Can you work these out from the model? Positions are in its coordinate system, mm. A direction names the side the tool comes from. Coordinates: 2 decimals unless noted, no trailing zeros. Loops run counter-clockwise (first coordinate to the right, second up) from the corner with the lowest first, then second, coordinate; pieces in that order, holes last.
Autodesk Inventor part; units mm, degrees
ref_plane "YZ Plane" through (0, 0, 0) normal (1, 0, 0) x (0, 1, 0)
ref_plane "XZ Plane" through (0, 0, 0) normal (0, 1, 0) x (-1, 0, 0)
ref_plane "XY Plane" through (0, 0, 0) normal (0, 0, 1) x (1, 0, 0)
sketch "Sketch1" plane through (0, 0, 0) normal (0, 0, 1) x (1, 0, 0)
  line L0 (185, -55) -> (-185, -55)
  line L1 (185, 55) -> (-185, 55)
  circle A0 centre (65, -25) radius 5.25
  line L2 (185, 55) -> (185, -55)
  line L3 (-185, 55) -> (-185, -55)
  line L4 (185, 55) -> (-185, -55) construction
  line L5 (185, -55) -> (-185, 55) construction
  line L6 (65, 25) -> (65, -25) construction
  line L7 (152.75, -30.25) -> (157.25, -30.25) construction
  line L8 (152.75, -35.5) -> (157.25, -35.5)
  line L9 (157.25, -25) -> (152.75, -25)
  arc A1 (152.75, -25) -> (152.75, -35.5) centre (152.75, -30.25) ccw
  arc A2 (157.25, -35.5) -> (157.25, -25) centre (157.25, -30.25) ccw
  line L10 (0, 0) -> (155, 0) construction
  line L11 (155, 0) -> (155, -30.25) construction
  dimension "d25" = 50
  dimension "d57" = 2.25
  dimension "d58" = 10.5
  dimension "d59" = 30.25
  dimension "d60" = 155
  dimension "d61" = 110
  dimension "d62" = 370
  dimension "d73" = 65
extrude "Plate1" add sketch "Sketch1" against normal blind 5 contours L0 L3 L1 L2 | A0 | A1 L9 A2 L8
sketch "Sketch4" plane through (185, 50, 0) normal (0, 1, 0) x (-1, 0, 0)
  line L0 (370, 0) -> (0, 0)
  line L1 (0, 0) -> (0, -40)
  line L2 (0, -40) -> (370, -40)
  line L3 (370, -40) -> (370, 0)
edge flange "Flange1" height 40 angle 90 thickness 5 bend radius 5 thickness toward (0, 1, 0) relief tear relief width 5 relief depth 2.5 corner gap 5 corner form 0 edges at (0, 55, -5) (0, -55, -5) wall of the first edge with corners at (-185, 50, 0) (185, 50, 0) (185, 50, -40) (-185, 50, -40)
bend "Bend3"
corner "Corner3"
extrude "Cut1" cut sketch "Sketch1" against normal blind 5 contours A1 L9 A2 L8
extrude "Cut2" cut sketch "Sketch1" against normal blind 5 contours A0
mirror "Mirror1" about plane through (0, 0, 0) normal (0, 1, 0) of "Cut2", "Cut1"
mirror "Mirror2" about plane through (0, 0, 0) normal (1, 0, 0) of "Cut2", "Cut1", "Mirror1"
equation "\"d74\" = Thickness"
equation "\"d76\" = Thickness"
equation "\"d78\" = Thickness"
equation "\"d63\" = BendReliefWidth"
equation "\"d64\" = BendReliefDepth"
equation "\"d65\" = MinimumRemnant"
equation "\"d66\" = BendRadius"
equation "\"d69\" = BendRadius"
equation "\"d70\" = CornerReliefSize"
equation "\"d71\" = GapSize"
equation "\"d72\" = JacobiRadiusSize"
equation "\"BendRadius\" = Thickness"
equation "\"BendReliefWidth\" = Thickness"
equation "\"BendReliefDepth\" = 0.5 * Thickness"
equation "\"TransitionRadius\" = BendRadius"
equation "\"JacobiRadiusSize\" = Thickness"
equation "\"d36\" = BendRadius"
equation "\"GapSize\" = Thickness"
properties part number "ADSK-MH-10032" material "Steel, Mild"
Item 1: I'm going to push flat-ended pins straight in: P1, Ø1.3, axis at x = -155, z = -2.5, coming from the +Y side; P2, Ø5, axis at x = 154.5, z = -3, coming from the +Y side; P3, Ø2, axis at x = -156, z = -2.5, coming from the -Y side. Where does each tip first touch, or does it pass through?
Results are:
P1: stops at y = 52.29
P2: stops at y = 53.93
P3: stops at y = -52.6
Item 2: Suppose I cut it at A-A, the plane z = -23. Please give me the cut outline in (x, y), plus the area to 3 significant figures.
Results are:
outline: (-185, -55) - (185, -55) - (185, -50) - (-185, -50) - close; (-185, 50) - (185, 50) - (185, 55) - (-185, 55) - close
area: 3,700 mm2
Item 3: Suppose I cut it at C-C, the plane x = -116.5. Please give me the cut outline in (y, z).
Results are:
outline: (-55, -40) - (-50, -40) - (-50, -10) arc R5 cw to (-45, -5) - (45, -5) arc R5 cw to (50, -10) - (50, -40) - (55, -40) - (55, -10) arc R10 ccw to (45, 0) - (-45, 0) arc R10 ccw to (-55, -10) - close
Item 4: On a 3-axis mill with a long thin cutter (end or side, diameter ignored), from which of +Z, -Z, +X, -X, +Y, -Y can I reach the whole of each face in a straight line? I mean faces 5 (the face through (-3, 1, -5)), 6 (the face through (-3, -55, -25)). Say none if no direction works.
Results are:
face 5: -Z, +X, -X
face 6: +Z, -Z, +X, -X, -Y
Item 5: Suppose I cut it at B-B, the plane x = 65. Please give me the cut outline in (y, z), plus the area to 3 significant figures.
Results are:
outline: (-55, -40) - (-50, -40) - (-50, -10) arc R5 cw to (-45, -5) - (-30.25, -5) - (-30.25, 0) - (-45, 0) arc R10 ccw to (-55, -10) - close; (-19.75, -5) - (19.75, -5) - (19.75, 0) - (-19.75, 0) - close; (30.25, -5) - (45, -5) arc R5 cw to (50, -10) - (50, -40) - (55, -40) - (55, -10) arc R10 ccw to (45, 0) - (30.25, 0) - close
area: 763 mm2
Item 6: I need wall thicknesses on line 1 along Y through (x, z) = (-65, -1.3); line 2 along Y through (x, z) = (118, -21); line 3 along Y through (x, z) = (65, -1). Which ranges of each line are inside material? Lowest first, please.
Results are:
line 1: y = -49.93 to -30.25, -19.75 to 19.75, 30.25 to 49.93
line 2: y = -55 to -50, 50 to 55
line 3: y = -49.36 to -30.25, -19.75 to 19.75, 30.25 to 49.36
Item 7: Suppose I cut it at D-D, the plane y = -9. Please give me the cut outline in (x, z).
Results are:
outline: (-185, -5) - (185, -5) - (185, 0) - (-185, 0) - close
Item 8: We'd pull the mould along X, two halves only. Please class faces 1 (the face through (-3, -50, -25)), 2 (the face through (-185, 0, -4)), 3 (the face through (60.83, 21.81, -2.46)), 4 (the face through (-60.83, -21.81, -2.46)): +X half, -X half, draft (parallel to the pull), parting line (faces both ways), or undercut.
Results are:
face 1: draft
face 2: -X half
face 3: undercut
face 4: undercut
